Work out the finished part from the listing and answer in its coordinate system (mm). A direction names the side the tool comes from. Coordinates: 2 decimals unless noted, no trailing zeros. Write each loop counter-clockwise with the first axis right and the second up, starting at its lowest first coordinate (ties: lowest second). Pieces come first, ordered by that corner, then holes. Notation, with made-up numbers: (-35.75, -10) - (23.25, -10) arc R27 cw to (23.25, 17) - close; hole circle Ø7 at (-23, 63.25). An arc over 180 degrees is marked (long way). One line per item, written item: value.
Autodesk Fusion 360 part; units mm, degrees
sketch "Sketch1" plane through (0, 0, 0) normal (0, 0, 1) x (1, 0, 0)
  line L0 (0, 0) -> (0, 20)
  line L1 (0, 20) -> (16, 20)
  line L2 (0, 0) -> (6, 0)
  line L3 (0, 0) -> (10, 0)
  line L4 (16, 20) -> (16, 6)
  line L5 (10, 0) -> (16, 6)
  dimension "d1" = 20
  dimension "d2" = 16
  dimension "d3" = 14
extrude "Extrude1" add sketch "Sketch1" along normal blind 6
sketch "Sketch2" plane through (0, 0, 6) normal (0, 0, 1) x (-1, 0, 0)
  line L0 (0, 0) -> (-10, 0)
  line L1 (-10, 0) -> (-16, -6)
  line L2 (-16, -6) -> (-16, -20)
  line L3 (-16, -20) -> (0, -20)
  line L4 (0, -20) -> (0, 0)
  line L5 (0, 0) -> (-2, 0)
  line L6 (-2, 0) -> (-2, -4)
  line L7 (0, 0) -> (0, -16)
  line L8 (0, -16) -> (-8, -16)
  line L9 (-8, -16) -> (-8, -10)
  line L10 (-2, -4) -> (-8, -10)
  dimension "d6" = 2
  dimension "d7" = 4
  dimension "d8" = 16
  dimension "d9" = 8
  dimension "d10" = 6
extrude "Extrude2" add sketch "Sketch2" along normal blind 4 contours L0 L4 L5 L6 L7 L8 L9 L10
sketch "Sketch3" plane through (0, 0, 6) normal (0, 0, 1) x (-1, 0, 0)
  line L0 (-2, -4) -> (-2, 0)
  line L1 (-2, 0) -> (-10, 0)
  line L2 (-10, 0) -> (-16, -6)
  line L3 (-16, -6) -> (-16, -20)
  line L4 (-16, -20) -> (0, -20)
  line L5 (0, -20) -> (0, -16)
  line L6 (0, -16) -> (-8, -16)
  line L7 (-8, -16) -> (-8, -10)
  line L8 (-8, -10) -> (-2, -4)
  line L9 (-16, -20) -> (-16, -18)
  line L10 (-8, -16) -> (-14, -16)
  line L11 (-14, -16) -> (-16, -18)
  line L12 (-16, -20) -> (0, -20)
  line L13 (0, -16) -> (0, -20)
  line L14 (0, -16) -> (-8, -16)
  dimension "d13" = 2
  dimension "d14" = 6
extrude "Extrude3" add sketch "Sketch3" along normal blind 6 contours L3 L4 L5 L6 L9 L10 L11 L12 L13 L14
sketch "Sketch4" plane through (0, 0, 10) normal (0, 0, 1) x (-1, 0, 0)
  line L0 (0, 0) -> (-2, 0)
  line L1 (-2, 0) -> (-2, -4)
  line L2 (-2, -4) -> (-8, -10)
  line L3 (-8, -10) -> (-8, -16)
  line L4 (-8, -16) -> (0, -16)
  line L5 (0, -16) -> (0, 0)
  line L6 (-8, -16) -> (-8, -13)
  line L7 (-8, -13) -> (-4, -13)
  dimension "d17" = 4
hole "Hole1" at (4, 13, 10) direction (0, 0, -1) diameter 2 depth 12 tip angle 118
sketch "Sketch5" plane through (0, 16, 0) normal (0, -1, 0) x (1, 0, 0)
  line L0 (0, 10) -> (8, 10)
  line L1 (8, 10) -> (8, 6)
  line L2 (8, 6) -> (14, 6)
  line L3 (14, 6) -> (14, 12)
  line L4 (14, 12) -> (0, 12)
  line L5 (0, 12) -> (0, 10)
  line L6 (14, 12) -> (11, 12)
  line L7 (11, 12) -> (11, 9)
  dimension "d21" = 3
  dimension "d22" = 3
hole "Hole2" at (11, 16, 9) direction (0, 1, 0) diameter 2 depth 12 tip angle 118
Item 1: Section D-D, the plane x = 6.25 is taken. Determine the outline of the cut face in (y, z), then the cut area to 3 significant figures.
Evaluation:
outline: (0, 0) - (20, 0) - (20, 12) - (16, 12) - (16, 10) - (8.25, 10) - (8.25, 6) - (0, 6) - close
area: 175 mm2
Item 2: Section B-B, the plane x = 4 is taken. Determine the outline of the cut face in (y, z), then the cut area to 3 significant figures.
Evaluation:
outline: (0, 0) - (12, 0) - (12, 10) - (6, 10) - (6, 6) - (0, 6) - close; (14, 0) - (20, 0) - (20, 12) - (16, 12) - (16, 10) - (14, 10) - close
area: 164 mm2
Item 3: Section A-A, the plane z = 9 is taken. Determine the outline of the cut face in (x, y), then the cut area to 3 significant figures.
Evaluation:
outline: (0, 0) - (2, 0) - (2, 4) - (8, 10) - (8, 16) - (10, 16) - (10, 20) - (0, 20) - close; (12, 16) - (14, 16) - (16, 18) - (16, 20) - (12, 20) - close; hole circle Ø2 at (4, 13)
area: 137 mm2
Item 4: Which of the six approach directions +Z, -Z, +X, -X, +Y, -Y give full straight-line access (tool end or side, diameter ignored) to faces 5 (the face through (2, 2, 8)), 6 (the face through (16, 13, 3))?
Evaluation:
face 5: +Z, +X, -Y
face 6: +Z, -Z, +X, +Y, -Y
Item 5: Given pin 1 (1.5 mm diameter, centred on x = 12, y = 4, fed in from +Z); pin 2 (2 mm diameter, centred on x = 9, y = 12.5, fed in from -Z); pin 3 (2.5 mm diameter, centred on x = 11, z = 9, fed in from -Y); pin 4 (9 mm diameter, centred on x = 3, y = 4, fed in from +Z), each flat-ended and moving along its own axis, determine where each tip first touches the part or whether it passes through.
Evaluation:
pin 1: stops at z = 6
pin 2: stops at z = 0
pin 3: stops at y = 16
pin 4: stops at z = 10
Item 6: Determine the mould class of faces 1 (the face through (3, 10, 10)), 2 (the face through (4, 0, 4)), 3 (the face through (4, 12, 5)), 4 (the face through (8, 20, 6)) for opening direction Y: +Y half, -Y half, draft (parallel to the pull), parting line (faces both ways), or undercut.
Evaluation:
face 1: draft
face 2: -Y half
face 3: undercut
face 4: +Y half
Item 7: Consider probe 1 along Y at (x, z) = (4, 4.25); probe 2 along X at (y, z) = (13, 5.5); probe 3 along X at (y, z) = (13, 6.25). Determine where each line is inside the solid, lowest interval first.
Evaluation:
probe 1: y = 0 to 12, 14 to 20
probe 2: x = 0 to 3, 5 to 16
probe 3: x = 0 to 3, 5 to 8
Item 8: Section C-C, the plane y = 17.5 is taken. Determine the outline of the cut face in (x, z), then the cut area to 3 significant figures.
Evaluation:
outline: (0, 0) - (16, 0) - (16, 6) - (15.5, 6) - (15.5, 12) - (0, 12) - close; hole circle Ø2 at (11, 9)
area: 186 mm2
